The figure shows three views and two pictorial views of one solid part (mm, origin at its lowest corner). Answer the questions. A direction names the side the tool comes from. Coordinates: 2 decimals unless noted, no trailing zeros. Loops run counter-clockwise (first coordinate to the right, second up) from the corner with the lowest first, then second, coordinate; pieces in that order, holes last. Notation, with made-up numbers: M 14.5,82 L 61.5,82 A25 ccw 61.5,111 Z; hole C -20.75,-36.75 d4. An arc over 180 degrees is marked long. Answer in a Markdown table with one row per item. Add a question column.
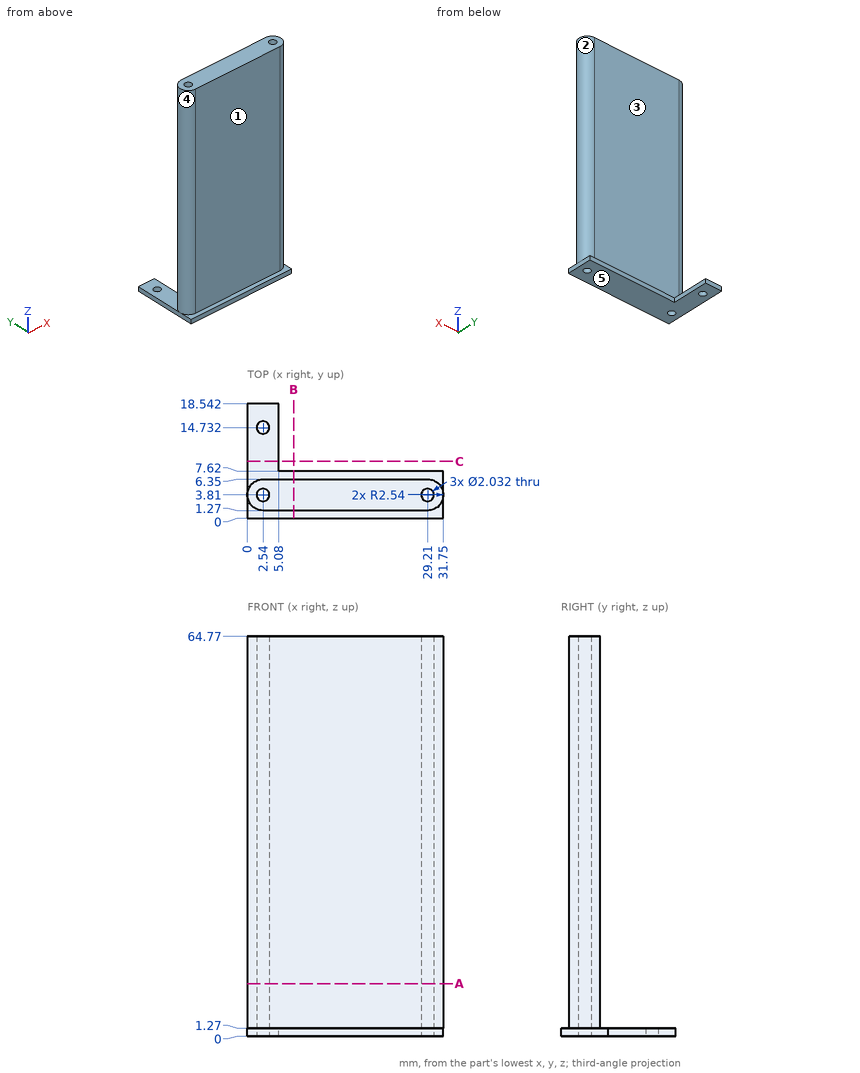
(1) A cutting plane is placed at C-C (y = 9.25). Give the vertices of the cut face in (x, z), plus the area to 3 significant figures.
(2) For the marked faces 1, 2, 3, 4 and 5, determine the directions among +Z, -Z, +X, -X, +Y, -Y from which every point of the face is accessible in a straight line to the end or side of a thin tool.
(3) A cutting plane is placed at B-B (x = 7.5). Give the vertices of the cut face in (y, z), plus the area to 3 significant figures.
(4) Each of these flat-tipped pins is pushed along its axis until it touches: pin 1 (4 mm diameter, centred on x = 19, z = 57, fed in from +Y); pin 2 (4 mm diameter, centred on y = 8, z = 38.5, fed in from +X); pin 3 (13.5 mm diameter, centred on x = 12.5, z = 17.5, fed in from -Y). Where does it stop, or does it pass through?
(5) A cutting plane is placed at A-A (z = 8.5). Give the vertices of the cut face in (x, y).
(6) Straight lines are drawn through the part: line 1 (Y direction, x = 2.54, z = 0.7); line 2 (X direction, y = 3, z = 22); line 3 (Y direction, x = 10, z = 43). For each, find the intervals that lie inside material, in ascending order.
Solved:
| question | item | result |
|---|---|---|
| 1 | outline | M 0,0 L 5.08,0 L 5.08,1.27 L 0,1.27 Z |
| 1 | area | 6.45 mm² |
| 2 | face 1 | +Z, +X, -X, -Y |
| 2 | face 2 | +Z, +X |
| 2 | face 3 | +Z, +X, -X, +Y |
| 2 | face 4 | +Z, -X |
| 2 | face 5 | -Z, +X, -X, +Y, -Y |
| 3 | outline | M 0,0 L 7.62,0 L 7.62,1.27 L 6.35,1.27 L 6.35,64.77 L 1.27,64.77 L 1.27,1.27 L 0,1.27 Z |
| 3 | area | 332 mm² |
| 4 | pin 1 | stops at y = 6.35 |
| 4 | pin 2 | stops at x = 30.5 |
| 4 | pin 3 | stops at y = 1.27 |
| 5 | outline | M 2.54,1.27 L 29.21,1.27 A2.54 ccw 29.21,6.35 L 2.54,6.35 A2.54 ccw Z; hole C 2.54,3.81 d2.03; hole C 29.21,3.81 d2.03 |
| 6 | line 1 | y = 0 to 2.79, 4.83 to 13.72, 15.75 to 18.54 |
| 6 | line 2 | x = 0.13 to 1.93, 3.15 to 28.6, 29.82 to 31.62 |
| 6 | line 3 | y = 1.27 to 6.35 |
